Study the drawing (mm; zero at the part's minimum x, y, z) and answer. A direction names the side the tool comes from. Round coordinates to 2 decimals unless told otherwise and drop trailing zeros. Write each loop counter-clockwise with the first axis right and the second up, starting at its lowest first coordinate (ties: lowest second). Pieces come first, ordered by that corner, then holes.
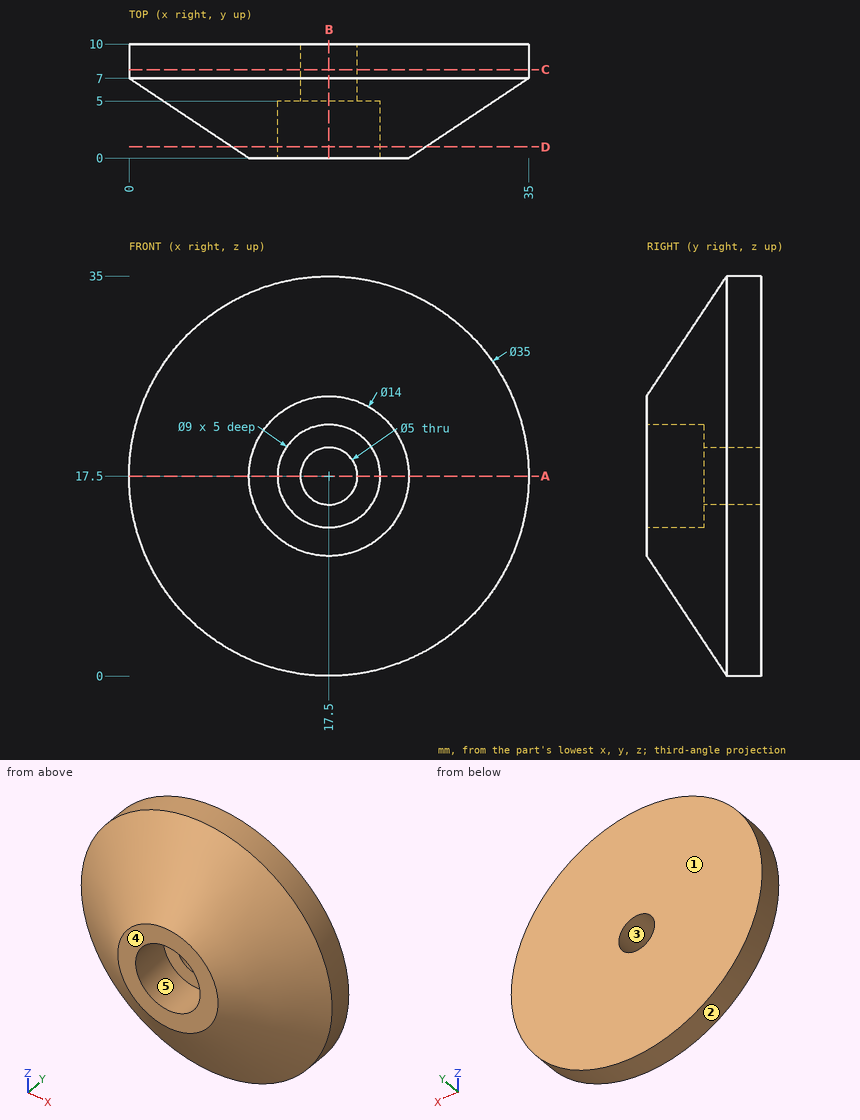
1. Section A-A on z = 17.5 is taken. Determine the outline of the cut face in (x, y).
Geometry says:
outline: (0, 7) - (10.5, 0) - (13, 0) - (13, 5) - (15, 5) - (15, 10) - (0, 10) - close; (20, 5) - (22, 5) - (22, 0) - (24.5, 0) - (35, 7) - (35, 10) - (20, 10) - close
2. For a pull along X with two mould halves and no side action, classify the marked faces 1, 2 and 3 as released by +X, released by -X, zero draft, split by the parting line, or undercut.
Geometry says:
face 1: zero draft
face 2: split by the parting line
face 3: undercut
3. Given pin 1 (4 mm diameter, centred on y = 7.5, z = 11.5, fed in from +X); pin 2 (4 mm diameter, centred on x = 6, y = 7.5, fed in from +Z); pin 3 (1.5 mm diameter, centred on x = 13.5, y = 2.5, fed in from -Z), each flat-ended and moving along its own axis, determine where each tip first touches the part or whether it passes through.
Geometry says:
pin 1: stops at x = 34.54
pin 2: stops at z = 32.2
pin 3: stops at z = 6.29
4. Section C-C on y = 7.75 is taken. Determine the outline of the cut face in (x, z), plus the area to 3 significant figures.
Geometry says:
outline: circle Ø35 at (17.5, 17.5); hole circle Ø5 at (17.5, 17.5)
area: 942 mm2
5. Straight lines are drawn through the part: line 1 along Z through (x, y) = (17.5, 7.85); line 2 along Y through (x, z) = (19, 21.5); line 3 along Z through (x, y) = (17.5, 6.2). For each, find the intervals that lie inside material, in ascending order.
Geometry says:
line 1: z = 0 to 15, 20 to 35
line 2: y = 5 to 10
line 3: z = 1.2 to 15, 20 to 33.8
6. Section D-D on y = 1 is taken. Determine the outline of the cut face in (x, z), plus the area to 3 significant figures.
Geometry says:
outline: circle Ø17 at (17.5, 17.5); hole circle Ø9 at (17.5, 17.5)
area: 163 mm2
7. Section B-B on x = 17.5 is taken. Determine the outline of the cut face in (y, z), plus the area to 4 significant figures.
Geometry says:
outline: (0, 10.5) - (7, 0) - (10, 0) - (10, 15) - (5, 15) - (5, 13) - (0, 13) - close; (0, 22) - (5, 22) - (5, 20) - (10, 20) - (10, 35) - (7, 35) - (0, 24.5) - close
area: 206.5 mm2
8. A tool of negligible diameter and unlimited length cuts with its end or side. For the marked faces 4 and 5, from which of +Z, -Z, +X, -X, +Y, -Y can it reach the whole face along a straight path? Write none if from no direction.
Geometry says:
face 4: +Z, -Z, +X, -X, -Y
face 5: -Y
